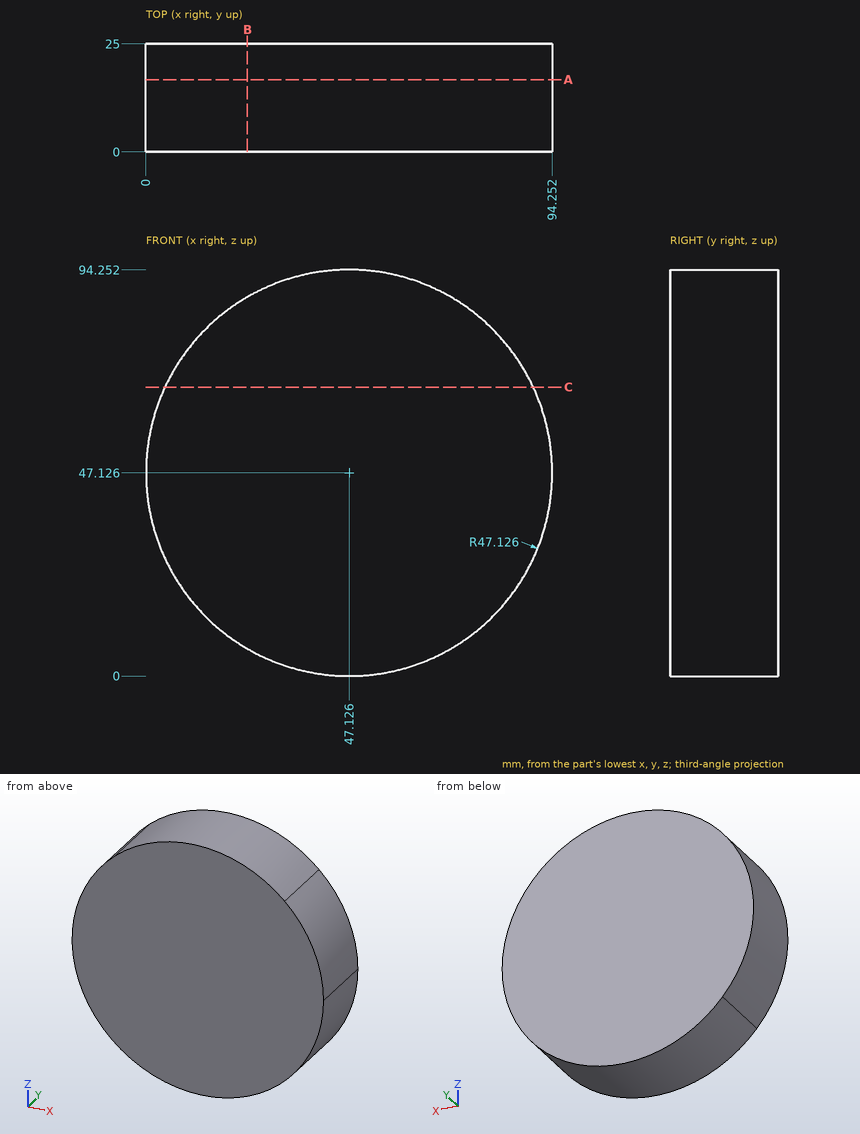
Input: dimensioned drawing with shaded views. Units: mm. Origin: part minimum x, y, z. Round coordinates to 2 decimals unless told otherwise and drop trailing zeros. Order: outer loops, then holes, each group sorted by start corner. A loop starts at its lowest first (then second) coordinate and runs counter-clockwise, first axis right, second up. Notation, with made-up numbers: (80.25, 18.25) - (135.25, 18.25) arc R17 ccw to (135.25, 47.25) - close; hole circle Ø7 at (-15, 25). An arc over 180 degrees is marked (long way). Answer as a JSON object with one key per item and string values. Group by question number.
(1) Cut plane B-B (x = 23.5). Return loops of the section in (y, z).
(2) Pin query (flat end, axial travel): P1, Ø6, axis at x = 56, y = 19, coming from the -Z side; P2, Ø3, axis at x = 22.5, y = 17, coming from the +Z side; P3, Ø1.5, axis at y = 5.5, z = 25.5, coming from the -X side. Return the tip coordinate at first contact, or that it passes through.
(3) Cut plane C-C (z = 67). Return loops of the section in (x, y).
(4) Cut plane A-A (y = 16.75). Return loops of the section in (x, z) (1 decimal), then the cut area to 3 significant figures.
(5) Material intervals for probe 1 along Z at (x, y) = (46.5, 2); probe 2 along Z at (x, y) = (10.5, 24); probe 3 along X at (y, z) = (24, 22) (1 decimal), sorted ascending. Write a range as from..to.
Here are the results:
{
 "1": {"outline": "(0, 6.35) - (25, 6.35) - (25, 87.9) - (0, 87.9) - close"},
 "2": {"P1": "stops at z = 0.37", "P2": "stops at z = 88.19", "P3": "stops at x = 4.88"},
 "3": {"outline": "(4.4, 0) - (89.86, 0) - (89.86, 25) - (4.4, 25) - close"},
 "4": {"outline": "(11.6, 16.1) arc R47.1 ccw to (81.2, 14.6) arc R47.1 ccw to (94.3, 47.1) arc R47.1 ccw to (79.7, 81.2) arc R47.1 ccw to (16.1, 82.6) arc R47.1 ccw to start", "area": "6,980 mm^2"},
 "5": {"probe 1": "z = 0..94.25", "probe 2": "z = 17.47..76.78", "probe 3": "x = 7.3..87"}
}
